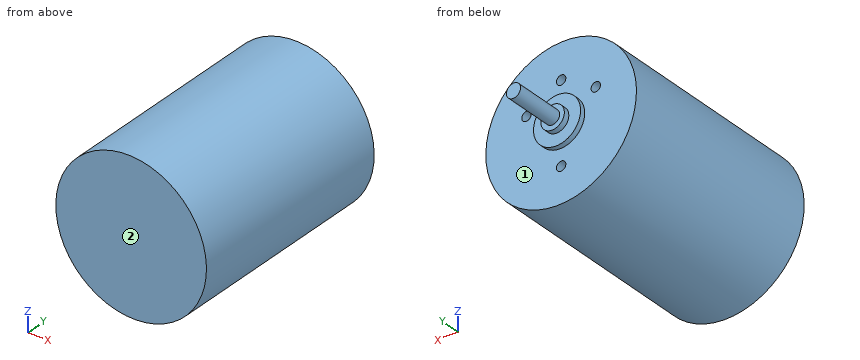
from build123d import *

# Parameters (mm, degrees)
SKETCH1_R           = 16
BOSS_EXTRUDE1_DEPTH = 45.05
SKETCH3_R           = 5
BOSS_EXTRUDE2_DEPTH = 1.1
SKETCH4_R           = 2.5
BOSS_EXTRUDE3_DEPTH = 1.2
SKETCH5_R           = 1.5
BOSS_EXTRUDE4_DEPTH = 10.5
SKETCH6_R           = 1
CUT_EXTRUDE1_DEPTH  = 3.6


with BuildPart() as part:
    # Sketch1 → Boss-Extrude1 (new body)
    with BuildSketch(Plane(origin=(0, 0, 0), x_dir=(1, 0, 0), z_dir=(0, 1, 0))):
        with Locations(Location((0, 0, 0), (0, 0, 270))):
            Circle(SKETCH1_R)
    extrude(amount=-BOSS_EXTRUDE1_DEPTH)

    # Sketch3 → Boss-Extrude2 (add)
    with BuildSketch(Plane(origin=(0, 0, 0), x_dir=(1, 0, 0), z_dir=(0, 1, 0))):
        with Locations(Location((0, 0, 0), (0, 0, 270))):
            Circle(SKETCH3_R)
    extrude(amount=BOSS_EXTRUDE2_DEPTH)

    # Sketch4 → Boss-Extrude3 (add)
    with BuildSketch(Plane(origin=(0, 1.1, 0), x_dir=(1, 0, 0), z_dir=(0, 1, 0))):
        with Locations(Location((0, 0, 0), (0, 0, 270))):
            Circle(SKETCH4_R)
    extrude(amount=BOSS_EXTRUDE3_DEPTH)

    # Sketch5 → Boss-Extrude4 (add)
    with BuildSketch(Plane(origin=(0, 2.3, 0), x_dir=(1, 0, 0), z_dir=(0, 1, 0))):
        with Locations(Location((0, 0, 0), (0, 0, 90))):
            Circle(SKETCH5_R)
    extrude(amount=BOSS_EXTRUDE4_DEPTH)

    # Sketch6 → Cut-Extrude1 (cut)
    with BuildSketch(Plane(origin=(0, 0, 0), x_dir=(1, 0, 0), z_dir=(0, 1, 0))):
        with Locations(Location((0, 8.5, 0), (0, 0, 270))):
            Circle(SKETCH6_R)
        with Locations(Location((0, -8.5, 0), (0, 0, 270))):
            Circle(SKETCH6_R)
        with Locations(Location((-7.361215932, -4.25, 0), (0, 0, 270))):
            Circle(SKETCH6_R)
        with Locations(Location((7.361215932, -4.25, 0), (0, 0, 270))):
            Circle(SKETCH6_R)
    extrude(amount=-CUT_EXTRUDE1_DEPTH, mode=Mode.SUBTRACT)


solid = part.part
Geometry check sheet. Reference: the model listing, model coordinates, mm. Face numbers are marked on the shaded views. A direction names the side the tool comes from. Round coordinates to 2 decimals unless told otherwise and drop trailing zeros. Order: outer loops, then holes, each group sorted by start corner. A loop starts at its lowest first (then second) coordinate and runs counter-clockwise, first axis right, second up. Notation, with made-up numbers: (49.5, -38.75) - (55.5, -38.75) arc R23 cw to (55.5, 0.25) - close; hole circle Ø1 at (-9, 69.25). An arc over 180 degrees is marked (long way). One line per question, with ' | ' between items. Start each with the question number.
(1) Sectioned sample at C-C on y = -29.5. Record the cut outline in (x, z).
(2) Sectioned sample at B-B on x = 0. Record the cut outline in (y, z), and give its area (3 significant figures).
(3) Sectioned sample at A-A on z = 0. Record the cut outline in (x, y).
(4) Access from +Z, -Z, +X, -X, +Y, -Y to the whole of each face (thin tool, end or side, straight path). Record for the marked faces 1 and 2.
(5) Thickness scan on L1, parallel to X at y = -2, z = 4; L2, parallel to Y at x = -11, z = 7; L3, parallel to X at y = -0.8, z = 8.5. Record the ranges inside material, lowest first. Write a range as [from, to].
(6) Depth check by flat-ended pin: pin 1 Ø4 at (x, y) = (5, -22) entering from +Z; pin 2 Ø2.5 at (x, z) = (-7.36, 4.25) entering from +Y; pin 3 Ø12 at (x, y) = (12.5, -4.5) entering from -Z. Enter the tip coordinate at first touch or a pass-through.
(7) Sectioned sample at D-D on z = 4.25. Record the cut outline in (x, y), and give its area (3 significant figures).
Conclusion:
1) outline: circle Ø32 at (0, 0)
2) outline: (-45.05, -16) - (0, -16) - (0, -9.5) - (-3.6, -9.5) - (-3.6, -7.5) - (0, -7.5) - (0, -5) - (1.1, -5) - (1.1, -2.5) - (2.3, -2.5) - (2.3, -1.5) - (12.8, -1.5) - (12.8, 1.5) - (2.3, 1.5) - (2.3, 2.5) - (1.1, 2.5) - (1.1, 5) - (0, 5) - (0, 7.5) - (-3.6, 7.5) - (-3.6, 9.5) - (0, 9.5) - (0, 16) - (-45.05, 16) - close | area: 1,480 mm2
3) outline: (-16, -45.05) - (16, -45.05) - (16, 0) - (5, 0) - (5, 1.1) - (2.5, 1.1) - (2.5, 2.3) - (1.5, 2.3) - (1.5, 12.8) - (-1.5, 12.8) - (-1.5, 2.3) - (-2.5, 2.3) - (-2.5, 1.1) - (-5, 1.1) - (-5, 0) - (-16, 0) - close
4) face 1: +Y | face 2: +Z, -Z, +X, -X, -Y
5) L1: x = [-15.49, -8.33], [-6.39, 6.39], [8.33, 15.49] | L2: y = [-45.05, 0] | L3: x = [-13.56, -1], [1, 13.56]
6) pin 1: stops at z = 15.72 | pin 2: stops at y = 0 | pin 3: stops at z = -14.62
7) outline: (-15.43, -45.05) - (15.43, -45.05) - (15.43, 0) - (8.36, 0) - (8.36, -3.6) - (6.36, -3.6) - (6.36, 0) - (2.63, 0) - (2.63, 1.1) - (-2.63, 1.1) - (-2.63, 0) - (-6.36, 0) - (-6.36, -3.6) - (-8.36, -3.6) - (-8.36, 0) - (-15.43, 0) - close | area: 1,380 mm2
